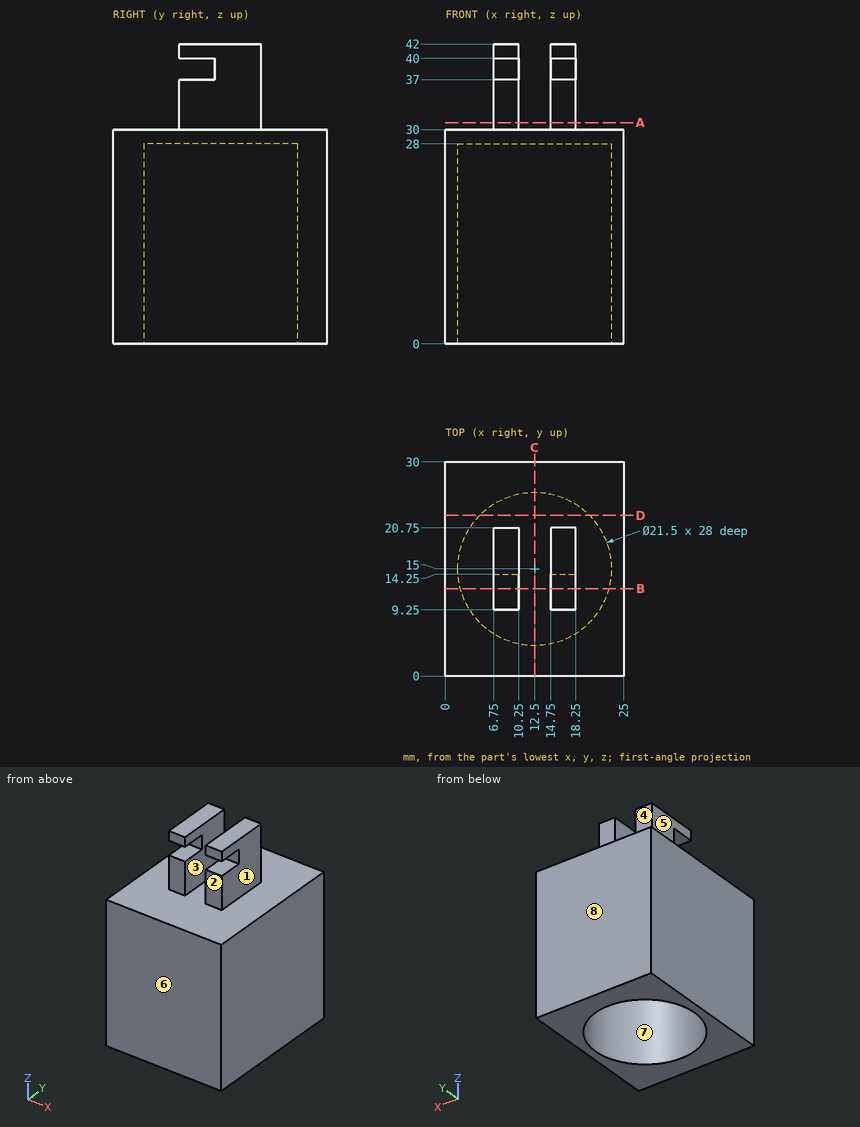
Job drawing, mm, ordinate dimensions from the low corner. One solid piece. A direction names the side the tool comes from. Give positions to 0.01 mm unless a question says otherwise; leave off trailing zeros. Order: outer loops, then holes, each group sorted by start corner. A loop starts at its lowest first (then second) coordinate and runs counter-clockwise, first axis right, second up. Notation, with made-up numbers: M 65,61 L 79,61 A25 cw 79,86 Z; hole C 73.5,-7.5 d9. An arc over 180 degrees is marked long. Put each result on its own line as item: value. Start each with the question number.
(1) Drill centre lines: L1, parallel to Y at x = 12.5, z = 15.5; L2, parallel to Z at x = 11.5, y = 4; L3, parallel to Z at x = 10.75, y = 8. Where is each one in solid material? Low to high. Write a range as [from, to].
(2) Pull direction Y, two halves, no side cores. Call the marked faces 6, 7 and 8: released by +Y, released by -Y, zero draft, split by the parting line, or undercut.
(3) Band-saw the part on D-D on y = 22.5. Give the cut face in (x, z), then the cut area to 3 significant figures.
(4) Band-saw the part on B-B on y = 12.25. Give the cut face in (x, z), then the cut area to 3 significant figures.
(5) Band-saw the part on A-A on z = 31. Give the cut face in (x, y).
(6) Tool access for the marked faces 1, 2, 3, 4 and 5: list every direction of +Z, -Z, +X, -X, +Y, -Y with a clear straight run to the whole face (end or side of a thin tool).
(7) Band-saw the part on C-C on x = 12.5. Give the cut face in (y, z).
(8) Pin check, flat tips, straight feed: pin 1 Ø1.8 at (x, y) = (16, 12.5) entering from -Z; pin 2 Ø2.5 at (x, z) = (8, 38.5) entering from -Y; pin 3 Ø2 at (x, z) = (16.5, 41) entering from -Y. Stop position of each tip, or through.
Results below:
1. L1: y = [0, 4.25], [25.75, 30]
1. L2: z = [0, 30]
1. L3: z = [28, 30]
2. face 6: released by -Y
2. face 7: undercut
2. face 8: released by +Y
3. outline: M 0,0 L 4.8,0 L 4.8,28 L 20.2,28 L 20.2,0 L 25,0 L 25,30 L 0,30 Z
3. area: 319 mm2
4. outline: M 0,0 L 2.11,0 L 2.11,28 L 22.89,28 L 22.89,0 L 25,0 L 25,30 L 18.25,30 L 18.25,37 L 14.75,37 L 14.75,30 L 10.25,30 L 10.25,37 L 6.75,37 L 6.75,30 L 0,30 Z; M 6.75,40 L 10.25,40 L 10.25,42 L 6.75,42 Z; M 14.75,40 L 18.25,40 L 18.25,42 L 14.75,42 Z
4. area: 231 mm2
5. outline: M 6.75,9.25 L 10.25,9.25 L 10.25,20.75 L 6.75,20.75 Z; M 14.75,9.25 L 18.25,9.25 L 18.25,20.75 L 14.75,20.75 Z
6. face 1: +Z, +X, +Y, -Y
6. face 2: +Z, +X, -X, -Y
6. face 3: +Z, +Y, -Y
6. face 4: +Z, +X, -X, +Y
6. face 5: +Z, -X, +Y, -Y
7. outline: M 0,0 L 4.25,0 L 4.25,28 L 25.75,28 L 25.75,0 L 30,0 L 30,30 L 0,30 Z
8. pin 1: stops at z = 28
8. pin 2: stops at y = 14.25
8. pin 3: stops at y = 9.25
